from build123d import *

# Parameters (mm, degrees)
F0_R     = 4.1275
F1_DEPTH = 3.175


# Not quite as in the source:
# - a feature names something its author has since deleted; it is built from what else it names


with BuildPart() as f1:
    # F0 (on Top) → F1 (new body)
    with BuildSketch(Plane.XY):
        with BuildLine():
            Line((81.1441976903, 48.870176137), (118.2163868425, 17.3270926481))
            ThreePointArc((118.2163868425, 17.3270926481), (125.7830950318, 15.1126819317), (133.6548019526, 14.6711869767))
            Line((133.6548019526, 14.6711869767), (347.9302216647, 27.1796528851))
            ThreePointArc((347.9302216647, 27.1796528851), (360.3982548534, 28.3159145983), (372.7658678172, 30.2614458507))
            Line((372.7658678172, 30.2614458507), (601.3625849364, 79.9327344304))
            ThreePointArc((601.3625849364, 79.9327344304), (611.9858366517, 85.4292367374), (618.4030760406, 95.5229998236))
            Line((618.4030760406, 95.5229998236), (632.5431455253, 176.5561104422))
            Line((632.5431455253, 176.5561104422), (636.893926966, 243.6304838067))
            ThreePointArc((636.893926966, 243.6304838067), (637.7262973987, 250.8582634049), (637.6190770743, 258.1330240374))
            Line((637.6190770743, 258.1330240374), (634.718536759, 294.5707376489))
            ThreePointArc((634.718536759, 294.5707376489), (634.0289947151, 313.0653425318), (634.89985466, 331.5522968769))
            Line((634.89985466, 331.5522968769), (639.2500827298, 410.037428213))
            ThreePointArc((639.2500827298, 410.037428213), (638.8544702471, 419.1155099086), (636.6822238963, 427.938741873))
            ThreePointArc((636.6822238963, 427.938741873), (634.7085093964, 431.5717815797), (631.6367376922, 434.3392253523))
            Line((631.6367376922, 434.3392253523), (567.6441777823, 474.7651219969))
            ThreePointArc((567.6441777823, 474.7651219969), (553.0816862682, 482.0654658914), (537.3700250266, 486.3671959048))
            Line((537.3700250266, 486.3671959048), (366.6023005126, 509.5713139182))
            ThreePointArc((366.6023005126, 509.5713139182), (356.5346140159, 510.2066384634), (346.480010855, 509.3899965888))
            Line((346.480010855, 509.3899965888), (192.7528221486, 489.8115695124))
            Line((192.7528221486, 489.8115695124), (99.3925322173, 475.4902721053))
            ThreePointArc((99.3925322173, 475.4902721053), (85.7762927803, 464.7559785435), (80.9017557977, 448.1166899806))
            Line((80.9017557977, 448.1166899806), (69.8140699742, 110.4154438382))
            ThreePointArc((69.8140699742, 110.4154438382), (71.8313111538, 86.8204891023), (74.6482450841, 63.3075982934))
            ThreePointArc((74.6482450841, 63.3075982934), (76.2705931102, 55.3574544062), (81.1441976903, 48.870176137))
        make_face()
        with Locations((125.2569147965, 27.2811080985)):
            Circle(F0_R, mode=Mode.SUBTRACT)
        with Locations((86.803833318, 59.6931402198)):
            Circle(F0_R, mode=Mode.SUBTRACT)
        with Locations((360.0400942892, 40.1343675154)):
            Circle(F0_R, mode=Mode.SUBTRACT)
        with Locations((598.7183749899, 99.1256637739)):
            Circle(F0_R, mode=Mode.SUBTRACT)
        with Locations((99.7337432835, 455.780702147)):
            Circle(F0_R, mode=Mode.SUBTRACT)
        with Locations((357.7462032552, 497.8582725917)):
            Circle(F0_R, mode=Mode.SUBTRACT)
        with Locations((619.9139634468, 418.3134020176)):
            Circle(F0_R, mode=Mode.SUBTRACT)
    extrude(amount=F1_DEPTH)


solid = f1.part
Source: CAD feature listing. Evaluate the final solid. Frame: model axes, mm. Coordinates: 2 decimals unless noted, no trailing zeros. Order: outer loops, then holes, each group sorted by start corner. A loop starts at its lowest first (then second) coordinate and runs counter-clockwise, first axis right, second up. Notation, with made-up numbers: M -37.75,-8 L -5.75,-8 A29 cw -5.75,18 Z; hole C 87,54 d4. An arc over 180 degrees is marked long. Write each question's results on one line, items separated by ' | '. Start each with the question number.
1. Section B-B, the plane x = 231.5. Return the cut outline in (y, z) (3 decimals), then the cut area to 3 significant figures.
2. Material intervals for L1, parallel to Y at x = 210, z = 0.9; L2, parallel to X at y = 191.5, z = 0.9; L3, parallel to X at y = 318, z = 2.35, sorted ascending.
3. Section C-C, the plane y = 120.5. Return the cut outline in (x, z) (1 decimal).
4. Section A-A, the plane z = 2.3. State how many separate pieces and enclosed holes the cut face has, then the cut area to 3 significant figures.
5. Pin query (flat end, axial travel): pin 1 (1 mm diameter, centred on y = 215, z = 2, fed in from -X); pin 2 (1.5 mm diameter, centred on x = 256, z = 2.5, fed in from -Y); pin 3 (1.5 mm diameter, centred on x = 555, z = 1.5, fed in from +Y). Return the tip coordinate at first contact, or that it passes through.
Solution:
1) outline: M 20.383,0 L 494.746,0 L 494.746,3.175 L 20.383,3.175 Z | area: 1,510 mm²
2) L1: 19.13 to 492.01 | L2: 72.48 to 633.51 | L3: 76.63 to 634.11
3) outline: M 70.1,0 L 622.8,0 L 622.8,3.2 L 70.1,3.2 Z
4) separate pieces: 1 | enclosed holes: 7 | area: 250,000 mm²
5) pin 1: x = 73.23 | pin 2: y = 21.77 | pin 3: y = 481.61
